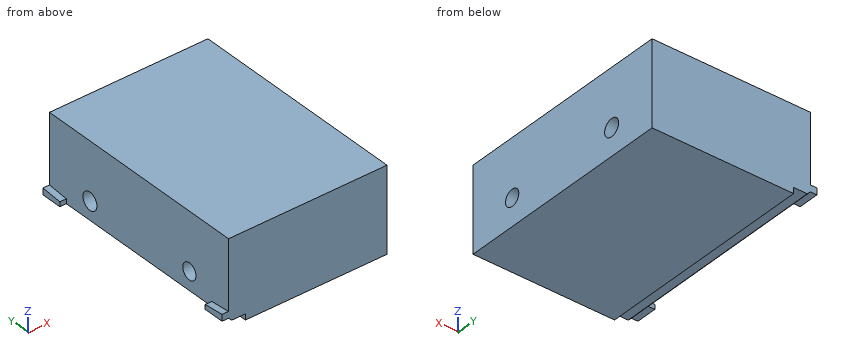
```python
from build123d import *

# Parameters (mm, degrees)
F0_W     = 77.47
F0_H     = 107.95
F1_DEPTH = 41.275
F2_R     = 3.9878
F2_R_2   = 4.2274185689
F3_DEPTH = 77.471
F5_DEPTH = 107.951
F7_DEPTH = 3.175


# Not quite as in the source:
# - a pattern or mirror of a feature is missing from the dataset's text; its kind, count and spacing are read off the source's solid


with BuildPart() as f1:
    # F0 (on Top) → F1 (new body)
    with BuildSketch(Plane.XY):
        Rectangle(F0_W, F0_H)
    extrude(amount=F1_DEPTH)

    # F2 (on face) → F3 (cut, through all)
    with BuildSketch(Plane.YZ.offset(38.735)):
        with Locations((-30.3550828248, 13.335)):
            Circle(F2_R)
        with Locations((29.6055749059, 13.335)):
            Circle(F2_R_2)
    extrude(amount=-F3_DEPTH, mode=Mode.SUBTRACT)

    # F4 (on face) → F5 (cut, through all)
    with BuildSketch(Plane(origin=(0, 53.975, 0), x_dir=(-1, 0, 0), z_dir=(0, 1, 0))):
        Polygon((38.735, 0), (38.735, 4.445), (37.1475, 2.8575), (30.48, 2.8575), (30.48, 0), align=None)
    extrude(amount=-F5_DEPTH, mode=Mode.SUBTRACT)

    # F6 (on face) → F7 (join)
    with BuildSketch(Plane(origin=(-38.735, 0, 0), x_dir=(0, -1, 0), z_dir=(-1, 0, 0))):
        Polygon((-53.975, 7.62), (-53.975, 4.445), (-43.815, 4.445), (-43.815, 6.7311151786), align=None)
    f7 = extrude(amount=F7_DEPTH)

    # F7_copies: F7 across plane
    add(f7.mirror(Plane(origin=(0, 0, 0), x_dir=(0, 0, -1), z_dir=(0, -1, 0))))


solid = f1.part
```
Geometry: final body of the model. Coordinates: model frame, mm. Give positions to 0.01 mm unless a question says otherwise; leave off trailing zeros. Loops run counter-clockwise (first coordinate to the right, second up) from the corner with the lowest first, then second, coordinate; pieces in that order, holes last. Notation, with made-up numbers: (75, -36) -> (99, -36) arc R23 cw to (99, -14) -> close; hole circle Ø7 at (60.25, 77). An arc over 180 degrees is marked (long way). Return JSON: item names as keys, results as strings.
Item 1: Line query: line 1 (Y direction, x = 34, z = 15) (1 decimal); line 2 (Z direction, x = 0.5, y = 29.5) (3 decimals); line 3 (Y direction, x = 10, z = 14) (3 decimals). Output: solid intervals per line, ascending.
Filled in:
{"line 1": "-54 to -34, -26.7 to 25.7, 33.5 to 54", "line 2": "0 to 9.109, 17.561 to 41.275", "line 3": "-53.975 to -34.287, -26.423 to 25.431, 33.78 to 53.975"}
Item 2: Section B-B, the plane y = -14. Output: boundary loops of the cut face in (x, z) (1 decimal), plus the area to 3 significant figures.
Filled in:
{"outline": "(-38.7, 4.4) -> (-37.1, 2.9) -> (-30.5, 2.9) -> (-30.5, 0) -> (38.7, 0) -> (38.7, 41.3) -> (-38.7, 41.3) -> close", "area": "3,170 mm^2"}
Item 3: Section A-A, the plane y = -33. Output: boundary loops of the cut face in (x, z) (1 decimal).
Filled in:
{"outline": "(-38.7, 4.4) -> (-37.1, 2.9) -> (-30.5, 2.9) -> (-30.5, 0) -> (38.7, 0) -> (38.7, 10.4) -> (-38.7, 10.4) -> close; (-38.7, 16.3) -> (38.7, 16.3) -> (38.7, 41.3) -> (-38.7, 41.3) -> close"}
Item 4: Section D-D, the plane z = 19. Output: boundary loops of the cut face in (x, y) (3 decimals).
Filled in:
{"outline": "(-38.735, -53.975) -> (38.735, -53.975) -> (38.735, 53.975) -> (-38.735, 53.975) -> close"}
Item 5: Section C-C, the plane x = -27. Output: boundary loops of the cut face in (y, z) (3 decimals), plus the area to 3 significant figures.
Filled in:
{"outline": "(-53.975, 0) -> (53.975, 0) -> (53.975, 41.275) -> (-53.975, 41.275) -> close; hole circle Ø7.976 at (-30.355, 13.335); hole circle Ø8.455 at (29.606, 13.335)", "area": "4,350 mm^2"}
Item 6: Pin query (flat end, axial travel): P1, Ø5, axis at y = -30.36, z = 13.34, coming from the -X side; P2, Ø1, axis at x = -40.5, y = -49.5, coming from the -Z side (3 decimals); P3, Ø5, axis at y = 31, z = 15, coming from the -X side (3 decimals); P4, Ø2, axis at x = -34.5, y = -9.5, coming from the -Z side. Return the tip coordinate at first contact, or that it passes through.
Filled in:
{"P1": "through", "P2": "z = 4.445", "P3": "x = -38.735", "P4": "z = 2.86"}
